Geometry: final body of the model. Coordinates: model frame, mm. Round coordinates to 2 decimals unless told otherwise and drop trailing zeros. Write each loop counter-clockwise with the first axis right and the second up, starting at its lowest first coordinate (ties: lowest second). Pieces come first, ordered by that corner, then holes. Notation, with made-up numbers: (-25.5, 21) -> (18.5, 21) arc R12 ccw to (18.5, 31) -> close; hole circle Ø1 at (-10, 28). An arc over 180 degrees is marked (long way). One line per item, written item: value. Start each with the question number.
from build123d import *

# Parameters (mm, degrees)
BOSS_EXTRU_1_DEPTH          = 5
ESQUISSE2_R                 = 5
ESQUISSE2_R_2               = 1.6
ENL_V_MAT_EXTRU_4_DEPTH     = 10
SYM_TRIE2_COPY_1_SKETCH_R   = 5
SYM_TRIE2_COPY_1_SKETCH_R_2 = 1.6
SYM_TRIE2_COPY_1_DEPTH      = 10


with BuildPart() as part:
    # Esquisse1 → Boss.-Extru.1 (new body)
    with BuildSketch(Plane(origin=(0, 0, 0), x_dir=(1, 0, 0), z_dir=(0, 1, 0))):
        Polygon((45, 87.5), (-70, 87.5), (-125, 87.5), (-125, 67.5), (-125, -67.5), (-125, -87.5), (-70, -87.5), (45, -87.5), (125, -87.5), (125, -42.5), (125, 42.5), (125, 87.5), align=None)
    extrude(amount=BOSS_EXTRU_1_DEPTH)

    # Esquisse2 → Enlèv. mat.-Extru.4 (cut)
    with BuildSketch(Plane(origin=(0, 5, 0), x_dir=(1, 0, 0), z_dir=(0, 1, 0))):
        with Locations(Location((85, -72, 0), (0, 0, 270))):
            Circle(ESQUISSE2_R)
        with Locations(Location((74.519765478, -62.717506566, 0), (0, 0, 270))):
            Circle(ESQUISSE2_R_2)
        with Locations(Location((74.519765478, -81.282493434, 0), (0, 0, 270))):
            Circle(ESQUISSE2_R_2)
        with Locations(Location((95.480234522, -81.282493434, 0), (0, 0, 270))):
            Circle(ESQUISSE2_R_2)
        with Locations(Location((95.480234522, -62.717506566, 0), (0, 0, 270))):
            Circle(ESQUISSE2_R_2)
    enl_v_mat_extru_4 = extrude(amount=-ENL_V_MAT_EXTRU_4_DEPTH, mode=Mode.SUBTRACT)

    # Symétrie1: Enlèv. mat.-Extru.4 across plane
    add(enl_v_mat_extru_4.mirror(Plane.XY), mode=Mode.SUBTRACT)

    # Symétrie2: Enlèv. mat.-Extru.4 across plane
    add(enl_v_mat_extru_4.mirror(Plane(origin=(0, 0, 0), x_dir=(0, 0, 1), z_dir=(1, 0, 0))), mode=Mode.SUBTRACT)

    # Symétrie2 copy 1 sketch → Symétrie2 copy 1 (cut)
    with BuildSketch(Plane(origin=(0, 5, 0), x_dir=(-1, 0, 0), z_dir=(0, 1, 0))):
        with Locations(Location((85, -72, 0), (0, 0, 270))):
            Circle(SYM_TRIE2_COPY_1_SKETCH_R)
        with Locations(Location((74.519765478, -62.717506566, 0), (0, 0, 270))):
            Circle(SYM_TRIE2_COPY_1_SKETCH_R_2)
        with Locations(Location((74.519765478, -81.282493434, 0), (0, 0, 270))):
            Circle(SYM_TRIE2_COPY_1_SKETCH_R_2)
        with Locations(Location((95.480234522, -81.282493434, 0), (0, 0, 270))):
            Circle(SYM_TRIE2_COPY_1_SKETCH_R_2)
        with Locations(Location((95.480234522, -62.717506566, 0), (0, 0, 270))):
            Circle(SYM_TRIE2_COPY_1_SKETCH_R_2)
    extrude(amount=-SYM_TRIE2_COPY_1_DEPTH, mode=Mode.SUBTRACT)


solid = part.part
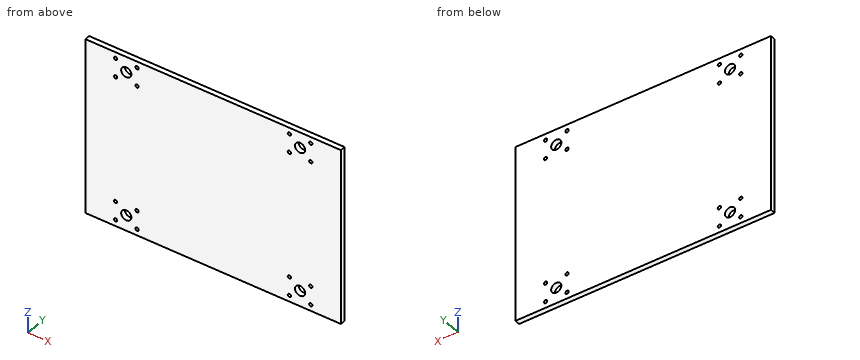
(1) Pin query (flat end, axial travel): pin 1 (2.5 mm diameter, centred on x = 74.52, z = -62.72, fed in from -Y). Return the tip coordinate at first contact, or that it passes through.
(2) Line query: probe 1 along X at (y, z) = (2.6, -72); probe 2 along X at (y, z) = (1.85, 70.5). Output: solid intervals per line, ascending.
(3) Section query A-A (z = -72). Output: boundary loops of the cut face in (x, y), and give its area (3 significant figures).
(4) Section query B-B (x = 85). Output: boundary loops of the cut face in (y, z), and give its area (3 significant figures).
Results list:
1. pin 1: passes through
2. probe 1: x = -125 to -90, -80 to 80, 90 to 125
2. probe 2: x = -125 to -89.77, -80.23 to 80.23, 89.77 to 125
3. outline: (-125, 0) -> (-90, 0) -> (-90, 5) -> (-125, 5) -> close; (-80, 0) -> (80, 0) -> (80, 5) -> (-80, 5) -> close; (90, 0) -> (125, 0) -> (125, 5) -> (90, 5) -> close
3. area: 1,150 mm^2
4. outline: (0, -87.5) -> (5, -87.5) -> (5, -77) -> (0, -77) -> close; (0, -67) -> (5, -67) -> (5, 67) -> (0, 67) -> close; (0, 77) -> (5, 77) -> (5, 87.5) -> (0, 87.5) -> close
4. area: 775 mm^2
